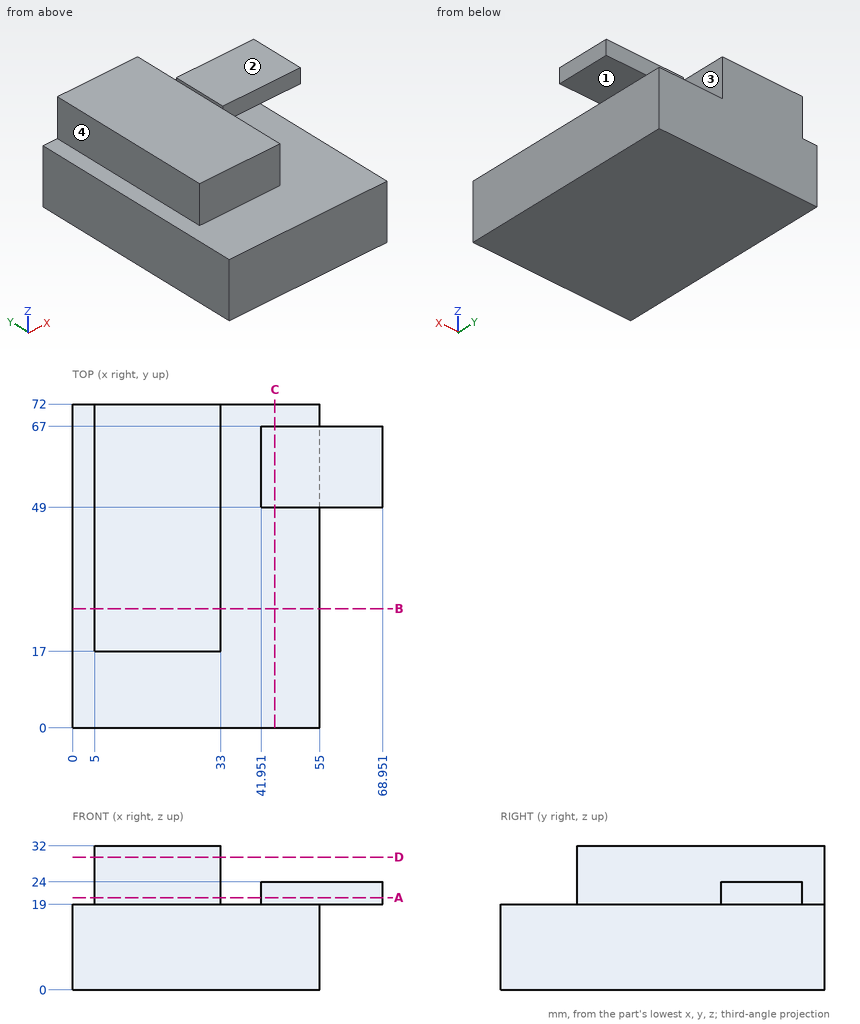
Study the drawing (mm; zero at the part's minimum x, y, z) and answer. A direction names the side the tool comes from. Give positions to 0.01 mm unless a question says otherwise; leave off trailing zeros. Write each loop counter-clockwise with the first axis right and the second up, starting at its lowest first coordinate (ties: lowest second). Pieces come first, ordered by that corner, then holes.
Item 1: Section B-B, the plane y = 26.5 is taken. Write down the section's boundary in (x, z).
Item 2: Section A-A, the plane z = 20.5 is taken. Write down the section's boundary in (x, y).
Item 3: Flat-ended cylindrical pins translate along their axes: P1, Ø10, axis at y = 32.5, z = 7.5, coming from the +X side; P2, Ø2.5, axis at y = 60.5, z = 22, coming from the -X side; P3, Ø5.5, axis at x = 53, y = 57, coming from the +Z side. Find the tip coordinate at first contact, or state that the pin passes through.
Item 4: Section D-D, the plane z = 29.5 is taken. Write down the section's boundary in (x, y).
Item 5: Find the intervals of material crossed by line 1 along X through (y, z) = (31, 15.5); line 2 along Z through (x, y) = (54, 44); line 3 along X through (y, z) = (24.5, 29), in increasing order.
Item 6: Which of the six approach directions +Z, -Z, +X, -X, +Y, -Y give full straight-line access (tool end or side, diameter ignored) to the marked faces 1, 2, 3 and 4?
Item 7: Section C-C, the plane x = 45 is taken. Write down the section's boundary in (y, z).
Completed:
1. outline: (0, 0) - (55, 0) - (55, 19) - (33, 19) - (33, 32) - (5, 32) - (5, 19) - (0, 19) - close
2. outline: (5, 17) - (33, 17) - (33, 72) - (5, 72) - close; (41.95, 49) - (68.95, 49) - (68.95, 67) - (41.95, 67) - close
3. P1: stops at x = 55
3. P2: stops at x = 5
3. P3: stops at z = 24
4. outline: (5, 17) - (33, 17) - (33, 72) - (5, 72) - close
5. line 1: x = 0 to 55
5. line 2: z = 0 to 19
5. line 3: x = 5 to 33
6. face 1: -Z, +X, +Y, -Y
6. face 2: +Z, +X, +Y, -Y
6. face 3: +Z, +Y, -Y
6. face 4: +Z, -X, +Y, -Y
7. outline: (0, 0) - (72, 0) - (72, 19) - (67, 19) - (67, 24) - (49, 24) - (49, 19) - (0, 19) - close
